```python
from build123d import *

# Parameters (mm, degrees)
SKETCH1_R             = 8
BOSS_EXTRUDE1_DEPTH   = 140
M8_TAPPED_HOLE1_D     = 6.8
M8_TAPPED_HOLE1_DEPTH = 19.75
M8_TAPPED_HOLE1_TIP   = 2.042926105
CHAMFER1_SIZE         = 1


with BuildPart() as part:
    # Sketch1 → Boss-Extrude1 (new body, symmetric)
    with BuildSketch(Plane(origin=(0, 0, 0), x_dir=(1, 0, 0), z_dir=(0, 1, 0))):
        Circle(SKETCH1_R)
    extrude(amount=BOSS_EXTRUDE1_DEPTH, both=True)

    # M8 Tapped Hole1
    with Locations(Plane(origin=(0, 140, 0), x_dir=(1, 0, 0), z_dir=(0, 1, 0))):
        with Locations((0, 0)):
            Hole(M8_TAPPED_HOLE1_D / 2, depth=M8_TAPPED_HOLE1_DEPTH)
            with Locations((0, 0, -(M8_TAPPED_HOLE1_DEPTH + M8_TAPPED_HOLE1_TIP / 2))):  # 118° drill point
                Cone(0, M8_TAPPED_HOLE1_D / 2, M8_TAPPED_HOLE1_TIP, mode=Mode.SUBTRACT)

    # Chamfer1
    chamfer1_edges = [part.edges().sort_by_distance(p)[0] for p in [
        (-8, 140, 0),
    ]]
    chamfer(chamfer1_edges, length=CHAMFER1_SIZE)


solid = part.part
```
Read the model definition and answer for the solid it produces. Units are mm, in the model's axes. Coordinates: 2 decimals unless noted, no trailing zeros. Write each loop counter-clockwise with the first axis right and the second up, starting at its lowest first coordinate (ties: lowest second). Pieces come first, ordered by that corner, then holes. Notation, with made-up numbers: (23, -34) -> (28, -34) arc R24 cw to (28, 3) -> close; hole circle Ø3 at (84, 65). An arc over 180 degrees is marked (long way). Write item = value, one per line.
(1) Given pin 1 Ø1 at (x, y) = (-4, 106) entering from -Z; pin 2 Ø3 at (y, z) = (-33.5, 2) entering from +X; pin 3 Ø4 at (x, y) = (2.5, 77) entering from -Z, each flat-ended and moving along its own axis, determine where each tip first touches the part or whether it passes through.
From the geometry:
pin_1 = -7.19
pin_2 = 7.98
pin_3 = -7.98
(2) For a pull along Z with two mould halves and no side action, classify faces 1 (the face through (0, -140, 0)), 2 (the face through (-0.128, 118.562, 0.576)), 3 (the face through (-1.73, 1.45, 7.81)), 4 (the face through (0.74, 129.99, 3.32)) as +Z half, -Z half, draft (parallel to the pull), parting line (faces both ways), or undercut.
From the geometry:
face_1 = draft
face_2 = undercut
face_3 = parting line
face_4 = undercut
(3) Section A-A on y = 6 is taken. Write down the section's boundary in (x, z).
From the geometry:
outline = circle Ø16 at (0, 0)
(4) Straight lines are drawn through the part: L1, parallel to Z at x = 0, y = 131.25; L2, parallel to Z at x = -0.5, y = 29; L3, parallel to Z at x = -2, y = -108. For each, find the intervals that lie inside material, in ascending order. Write a range as from..to.
From the geometry:
L1 = -8..-3.4, 3.4..8
L2 = -7.98..7.98
L3 = -7.75..7.75
